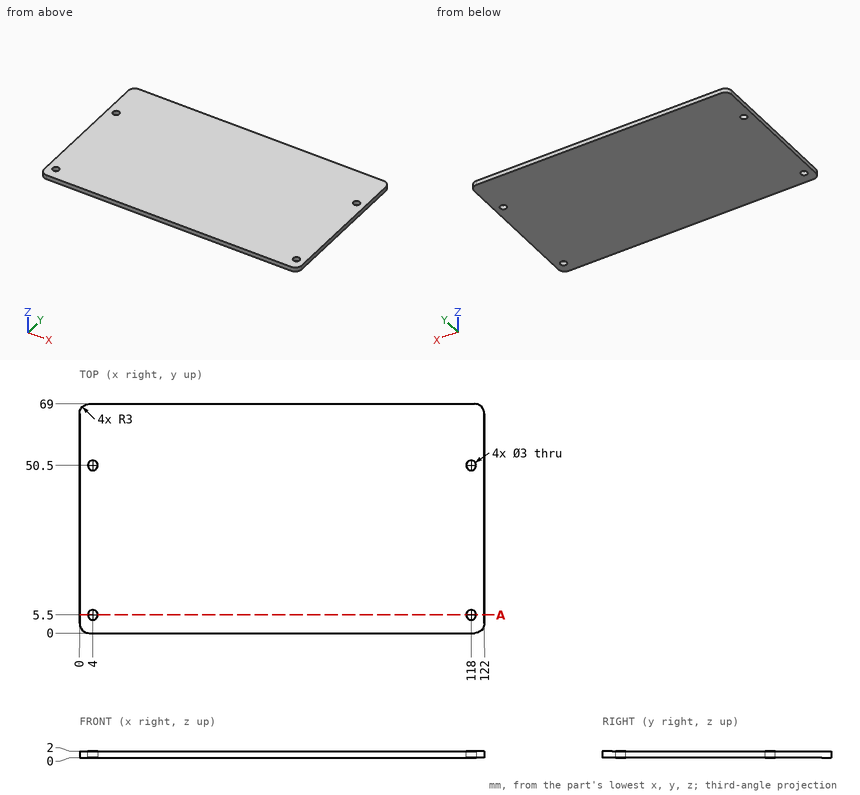
The figure shows three views and two pictorial views of one solid part (mm, origin at its lowest corner). Answer the questions. Give positions to 0.01 mm unless a question says otherwise; leave off trailing zeros. Order: outer loops, then holes, each group sorted by start corner. A loop starts at its lowest first (then second) coordinate and runs counter-clockwise, first axis right, second up. Notation, with made-up numbers: (-14, 55.25) -> (-3, 55.25) arc R17 cw to (-3, 70.25) -> close; hole circle Ø5 at (-4, 16.5). An arc over 180 degrees is marked (long way). Answer as CSV lines item,"result". Start each with the question number.
Q1. Given pin 1 (2.5 mm diameter, centred on x = 118, y = 5.5, fed in from +Z), flat-ended and moving along its own axis, determine where the tip first touches the part or whether it passes through.
Q2. A cutting plane is placed at A-A (y = 5.5). Determine the outline of the cut face in (x, z), then the cut area to 3 significant figures.
Q3. Find the intervals of material crossed by L1, parallel to Y at x = 118, z = 1.4; L2, parallel to X at y = 50, z = 0.2, in increasing order.
Results found:
1,pin 1,"through"
2,outline,"(0, 0) -> (2.5, 0) -> (2.5, 2) -> (0, 2) -> close; (5.5, 0) -> (116.5, 0) -> (116.5, 2) -> (5.5, 2) -> close; (119.5, 0) -> (122, 0) -> (122, 2) -> (119.5, 2) -> close"
2,area,"232 mm2"
3,L1,"0 to 4, 7 to 49, 52 to 69"
3,L2,"0 to 2.59, 5.41 to 116.59, 119.41 to 122"
